Answer from the drawing. Dimensions are ordinates in mm from the lowest x, y and z of the part. A direction names the side the tool comes from. Coordinates: 2 decimals unless noted, no trailing zeros. Write each loop counter-clockwise with the first axis right and the second up, starting at its lowest first coordinate (ties: lowest second). Pieces come first, ordered by that corner, then holes.
(1) The part is cut by section A-A, the plane x = 2.5. Determine the outline of the cut face in (y, z).
(2) Straight lines are drawn through the part: line 1 along Y through (x, z) = (55.5, 0.75); line 2 along X through (y, z) = (3, 0.55); line 3 along X through (y, z) = (31, 4.25). For each, find the intervals that lie inside material, in ascending order.
(3) The part is cut by section C-C, the plane y = 17.5. Determine the outline of the cut face in (x, z).
(4) Which of the six approach directions +Z, -Z, +X, -X, +Y, -Y give full straight-line access (tool end or side, diameter ignored) to the marked faces 1 and 2?
(5) The part is cut by section D-D, the plane z = 3.2. Determine the outline of the cut face in (x, y), and give its area (3 significant figures).
(6) Given pin 1 (2 mm diameter, centred on y = 9.5, z = 4, fed in from +X); pin 2 (3 mm diameter, centred on x = 2.5, y = 32.5, fed in from +Z); pin 3 (2.5 mm diameter, centred on y = 15, z = 3.5, fed in from -X); pin 4 (1.2 mm diameter, centred on x = 55.5, y = 2.5, fed in from -Z), each flat-ended and moving along its own axis, determine where each tip first touches the part or whether it passes through.
(7) The part is cut by section B-B, the plane y = 2.5. Determine the outline of the cut face in (x, z).
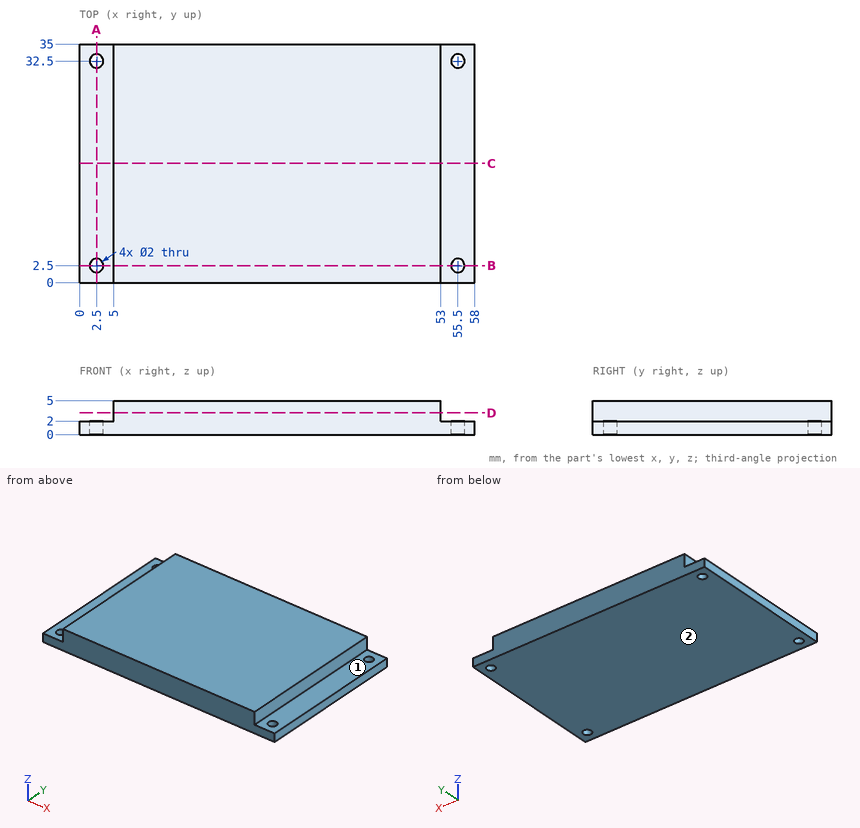
Computed:
1. outline: (0, 0) - (1.5, 0) - (1.5, 2) - (0, 2) - close; (3.5, 0) - (31.5, 0) - (31.5, 2) - (3.5, 2) - close; (33.5, 0) - (35, 0) - (35, 2) - (33.5, 2) - close
2. line 1: y = 0 to 1.5, 3.5 to 31.5, 33.5 to 35
2. line 2: x = 0 to 1.63, 3.37 to 54.63, 56.37 to 58
2. line 3: x = 5 to 53
3. outline: (0, 0) - (58, 0) - (58, 2) - (53, 2) - (53, 5) - (5, 5) - (5, 2) - (0, 2) - close
4. face 1: +Z, +X, +Y, -Y
4. face 2: -Z, +X, -X, +Y, -Y
5. outline: (5, 0) - (53, 0) - (53, 35) - (5, 35) - close
5. area: 1,680 mm2
6. pin 1: stops at x = 53
6. pin 2: stops at z = 2
6. pin 3: stops at x = 5
6. pin 4: passes through
7. outline: (0, 0) - (1.5, 0) - (1.5, 2) - (0, 2) - close; (3.5, 0) - (54.5, 0) - (54.5, 2) - (53, 2) - (53, 5) - (5, 5) - (5, 2) - (3.5, 2) - close; (56.5, 0) - (58, 0) - (58, 2) - (56.5, 2) - close
